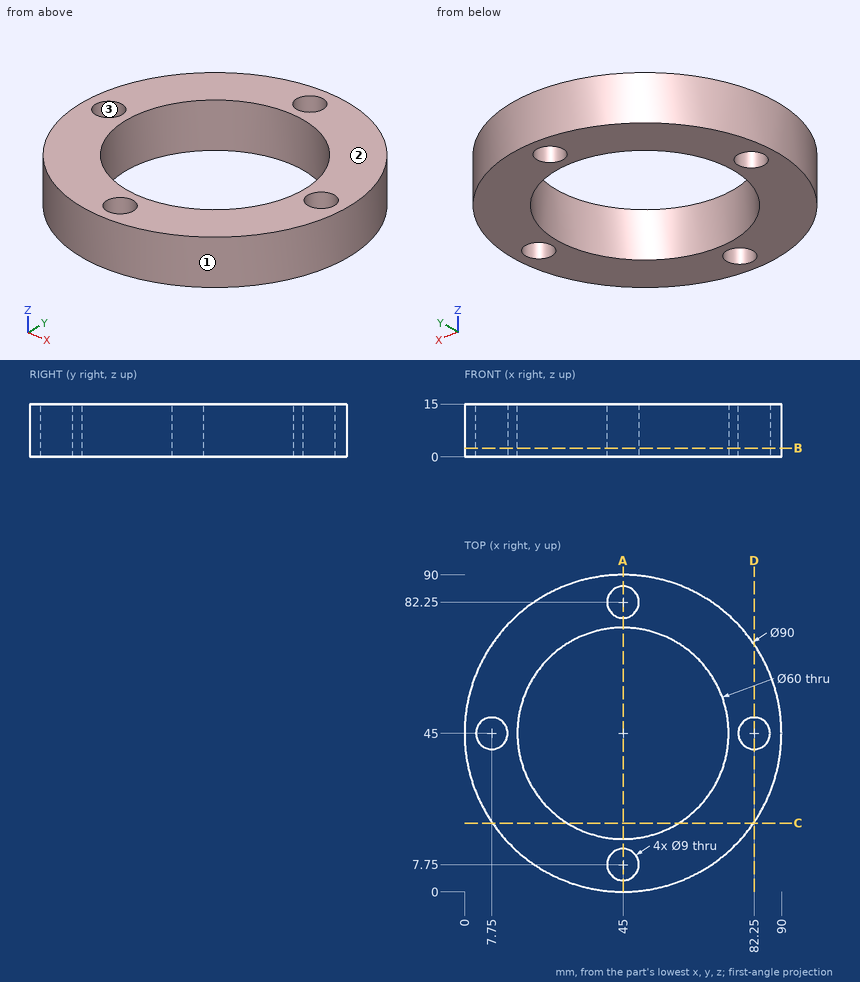
Geometry check sheet. Reference: drawing and pictorial views, mm from the part's lowest x, y, z. Give positions to 0.01 mm unless a question says otherwise; leave off trailing zeros. Write each loop counter-clockwise with the first axis right and the second up, starting at its lowest first coordinate (ties: lowest second). Pieces come first, ordered by that corner, then holes. Notation, with made-up numbers: (-8.75, -33) - (2.25, -33) arc R27 cw to (2.25, -12) - close; hole circle Ø9 at (71, 48.5). An arc over 180 degrees is marked (long way). Put each result on its own line as item: value.
Q1. Depth check by flat-ended pin: P1, Ø1.5, axis at y = 16.5, z = 4.5, coming from the -X side; P2, Ø5, axis at x = 59.5, z = 10, coming from the -Y side; P3, Ø1.5, axis at x = 47.5, z = 2, coming from the -Y side. Enter the tip coordinate at first touch or a pass-through.
Result:
P1: x = 9.57
P2: y = 1.63
P3: y = 0.03
Q2. Scan lines: probe 1 along Y at (x, z) = (45, 9.75); probe 2 along X at (y, z) = (47.5, 1.5); probe 3 along Y at (x, z) = (65, 9.75). Record each from-to range of solid material in increasing order. Write a range as from..to.
Result:
probe 1: 0..3.25, 12.25..15, 75..77.75, 86.75..90
probe 2: 0.07..4.01, 11.49..15.1, 74.9..78.51, 85.99..89.93
probe 3: 4.69..22.64, 67.36..85.31
Q3. Section check C-C on y = 19.5. Record the cut outline in (x, z), and give its area (3 significant figures).
Result:
outline: (7.92, 0) - (29.2, 0) - (29.2, 15) - (7.92, 15) - close; (60.8, 0) - (82.08, 0) - (82.08, 15) - (60.8, 15) - close
area: 638 mm2
Q4. Section check D-D on x = 82.25. Record the cut outline in (y, z).
Result:
outline: (19.75, 0) - (40.5, 0) - (40.5, 15) - (19.75, 15) - close; (49.5, 0) - (70.25, 0) - (70.25, 15) - (49.5, 15) - close
Q5. Section check B-B on z = 2.5. Record the cut outline in (x, y), and give its area (3 significant figures).
Result:
outline: circle Ø90 at (45, 45); hole circle Ø9 at (7.75, 45); hole circle Ø60 at (45, 45); hole circle Ø9 at (45, 7.75); hole circle Ø9 at (45, 82.25); hole circle Ø9 at (82.25, 45)
area: 3,280 mm2
Q6. Section check A-A on x = 45. Record the cut outline in (y, z), and give its area (3 significant figures).
Result:
outline: (0, 0) - (3.25, 0) - (3.25, 15) - (0, 15) - close; (12.25, 0) - (15, 0) - (15, 15) - (12.25, 15) - close; (75, 0) - (77.75, 0) - (77.75, 15) - (75, 15) - close; (86.75, 0) - (90, 0) - (90, 15) - (86.75, 15) - close
area: 180 mm2
Q7. Mould release check, pull along X, two halves, no side actions. Record for the marked faces 1, 2 and 3: released by +X, released by -X, zero draft, split by the parting line, or undercut.
Result:
face 1: split by the parting line
face 2: zero draft
face 3: undercut
